```python
from build123d import *

# Parameters (mm, degrees)
F0_R     = 2.1
F1_DEPTH = 500


with BuildPart() as f1:
    # F0 (on Top) → F1 (new body)
    with BuildSketch(Plane.XY):
        with BuildLine():
            Line((4.64, -10), (8.5, -10))
            Line((8.5, -10), (11.5, -10))
            Line((11.5, -10), (15.36, -10))
            Line((15.36, -10), (17.16, -8.2))
            Line((17.16, -8.2), (14.50066, -8.2))
            Line((14.50066, -8.2), (14.50066, -6.56))
            Line((14.50066, -6.56), (17.16, -3.90066))
            Line((17.16, -3.90066), (19.75, -3.90066))
            Line((19.75, -3.90066), (20, -3.65066))
            Line((20, -3.65066), (20.25, -3.90066))
            Line((20.25, -3.90066), (22.84, -3.90066))
            Line((22.84, -3.90066), (25.49934, -6.56))
            Line((25.49934, -6.56), (25.49934, -8.2))
            Line((25.49934, -8.2), (22.84, -8.2))
            Line((22.84, -8.2), (24.64, -10))
            Line((24.64, -10), (28.5, -10))
            ThreePointArc((28.5, -10), (29.56066, -9.56066), (30, -8.5))
            Line((30, -8.5), (30, -4.64))
            Line((30, -4.64), (28.2, -2.84))
            Line((28.2, -2.84), (28.2, -5.49934))
            Line((28.2, -5.49934), (26.56, -5.49934))
            Line((26.56, -5.49934), (23.90066, -2.84))
            Line((23.90066, -2.84), (23.90066, -0.25))
            Line((23.90066, -0.25), (23.65066, 0))
            Line((23.65066, 0), (23.90066, 0.25))
            Line((23.90066, 0.25), (23.90066, 2.84))
            Line((23.90066, 2.84), (26.56, 5.49934))
            Line((26.56, 5.49934), (28.2, 5.49934))
            Line((28.2, 5.49934), (28.2, 2.84))
            Line((28.2, 2.84), (30, 4.64))
            Line((30, 4.64), (30, 8.5))
            ThreePointArc((30, 8.5), (29.56066, 9.56066), (28.5, 10))
            Line((28.5, 10), (24.64, 10))
            Line((24.64, 10), (22.84, 8.2))
            Line((22.84, 8.2), (25.49934, 8.2))
            Line((25.49934, 8.2), (25.49934, 6.56))
            Line((25.49934, 6.56), (22.84, 3.90066))
            Line((22.84, 3.90066), (20.25, 3.90066))
            Line((20.25, 3.90066), (20, 3.65066))
            Line((20, 3.65066), (19.75, 3.90066))
            Line((19.75, 3.90066), (17.16, 3.90066))
            Line((17.16, 3.90066), (14.50066, 6.56))
            Line((14.50066, 6.56), (14.50066, 8.2))
            Line((14.50066, 8.2), (17.16, 8.2))
            Line((17.16, 8.2), (15.36, 10))
            Line((15.36, 10), (11.5, 10))
            Line((11.5, 10), (8.5, 10))
            Line((8.5, 10), (4.64, 10))
            Line((4.64, 10), (2.84, 8.2))
            Line((2.84, 8.2), (5.49934, 8.2))
            Line((5.49934, 8.2), (5.49934, 6.56))
            Line((5.49934, 6.56), (2.84, 3.90066))
            Line((2.84, 3.90066), (0.25, 3.90066))
            Line((0.25, 3.90066), (0, 3.65066))
            Line((0, 3.65066), (-0.25, 3.90066))
            Line((-0.25, 3.90066), (-2.84, 3.90066))
            Line((-2.84, 3.90066), (-5.49934, 6.56))
            Line((-5.49934, 6.56), (-5.49934, 8.2))
            Line((-5.49934, 8.2), (-2.84, 8.2))
            Line((-2.84, 8.2), (-4.64, 10))
            Line((-4.64, 10), (-8.5, 10))
            ThreePointArc((-8.5, 10), (-9.56066, 9.56066), (-10, 8.5))
            Line((-10, 8.5), (-10, 4.64))
            Line((-10, 4.64), (-8.2, 2.84))
            Line((-8.2, 2.84), (-8.2, 5.49934))
            Line((-8.2, 5.49934), (-6.56, 5.49934))
            Line((-6.56, 5.49934), (-3.90066, 2.84))
            Line((-3.90066, 2.84), (-3.90066, 0.25))
            Line((-3.90066, 0.25), (-3.65066, 0))
            Line((-3.65066, 0), (-3.90066, -0.25))
            Line((-3.90066, -0.25), (-3.90066, -2.84))
            Line((-3.90066, -2.84), (-6.56, -5.49934))
            Line((-6.56, -5.49934), (-8.2, -5.49934))
            Line((-8.2, -5.49934), (-8.2, -2.84))
            Line((-8.2, -2.84), (-10, -4.64))
            Line((-10, -4.64), (-10, -8.5))
            ThreePointArc((-10, -8.5), (-9.56066, -9.56066), (-8.5, -10))
            Line((-8.5, -10), (-4.64, -10))
            Line((-4.64, -10), (-2.84, -8.2))
            Line((-2.84, -8.2), (-5.49934, -8.2))
            Line((-5.49934, -8.2), (-5.49934, -6.56))
            Line((-5.49934, -6.56), (-2.84, -3.90066))
            Line((-2.84, -3.90066), (-0.25, -3.90066))
            Line((-0.25, -3.90066), (0, -3.65066))
            Line((0, -3.65066), (0.25, -3.90066))
            Line((0.25, -3.90066), (2.84, -3.90066))
            Line((2.84, -3.90066), (5.49934, -6.56))
            Line((5.49934, -6.56), (5.49934, -8.2))
            Line((5.49934, -8.2), (2.84, -8.2))
            Line((2.84, -8.2), (4.64, -10))
        make_face()
        Polygon((-6.56934, -7.63), (-6.56934, -8.2), (-8.2, -8.2), (-8.2, -6.56934), (-7.63, -6.56934), align=None, mode=Mode.SUBTRACT)
        Polygon((27.63, -6.56934), (28.2, -6.56934), (28.2, -8.2), (26.56934, -8.2), (26.56934, -7.63), align=None, mode=Mode.SUBTRACT)
        Circle(F0_R, mode=Mode.SUBTRACT)
        Polygon((-7.63, 6.56934), (-8.2, 6.56934), (-8.2, 8.2), (-6.56934, 8.2), (-6.56934, 7.63), align=None, mode=Mode.SUBTRACT)
        Polygon((3.90066, 2.84), (6.56, 5.49934), (6.99934, 5.93868), (6.99934, 8.2), (13.00066, 8.2), (13.00066, 5.93868), (13.44, 5.49934), (16.09934, 2.84), (16.09934, 0.25), (16.34934, 0), (16.09934, -0.25), (16.09934, -2.84), (13.44, -5.49934), (13.00066, -5.93868), (13.00066, -8.2), (6.99934, -8.2), (6.99934, -5.93868), (6.56, -5.49934), (3.90066, -2.84), (3.90066, -0.25), (3.65066, 0), (3.90066, 0.25), align=None, mode=Mode.SUBTRACT)
        with Locations((20, 0)):
            Circle(F0_R, mode=Mode.SUBTRACT)
        Polygon((28.2, 8.2), (28.2, 6.56934), (27.63, 6.56934), (26.56934, 7.63), (26.56934, 8.2), align=None, mode=Mode.SUBTRACT)
    extrude(amount=F1_DEPTH)


solid = f1.part
```
Can you work these out from the model? Positions are in its coordinate system, mm. Give positions to 0.01 mm unless a question says otherwise; leave off trailing zeros. Write item = value, one per line. Start each with the question number.
1. Imagine slicing it at A-A (z = 222). Count the separate pieces of the cut face and the enclosed holes in it, and give its area (3 significant figures).
2. For pin 1 (0.8 mm diameter, centred on y = 2, z = 234.5, fed in from -X); pin 2 (2 mm diameter, centred on y = -2, z = 360.5, fed in from -X); pin 3 (0.8 mm diameter, centred on x = -4, z = 260, fed in from +Y), each with a flat end and sliding along its axis, tell me the tip position at first contact or that it passes through.
3. Please list where these lines run through material, in increasing order: line 1 (X direction, y = -0.25, z = 264); line 2 (X direction, y = 6.5, z = 390); line 3 (X direction, y = -7.75, z = 304.5).
Worked answers:
q1.separate_pieces = 1
q1.enclosed_holes = 7
q1.area = 287 mm2
q2.pin_1 = -3.9
q2.pin_2 = -8.36
q2.pin_3 = 9.76
q3.line_1 = -3.9 to -2.09, 2.09 to 3.9, 16.1 to 17.91, 22.09 to 23.9
q3.line_2 = -10 to -5.44, 5.44 to 7, 13 to 14.56, 25.44 to 30
q3.line_3 = -10 to -8.2, -6.57 to -5.5, 5.5 to 7, 13 to 14.5, 25.5 to 26.57, 28.2 to 30
